Source: three-view drawing plus pictorial views. Frame: mm from the lowest corner of the part. A direction names the side the tool comes from. Give positions to 0.01 mm unless a question says otherwise; leave off trailing zeros. Order: outer loops, then holes, each group sorted by start corner. A loop starts at its lowest first (then second) coordinate and runs counter-clockwise, first axis right, second up. Notation, with made-up numbers: (24.25, 10) -> (83.25, 10) arc R27 cw to (83.25, 28) -> close; hole circle Ø8 at (86, 9.5). An arc over 180 degrees is marked (long way). One line per question, with ' | ' between items.
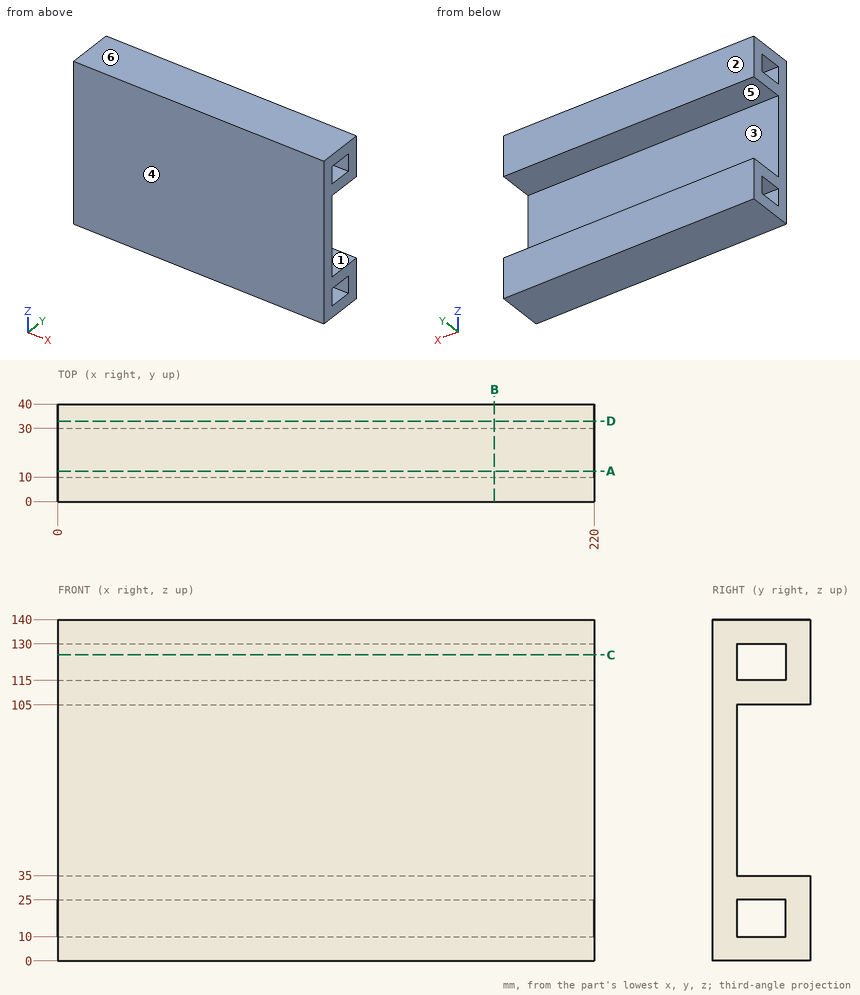
1) Section B-B on x = 179. Return loops of the section in (y, z).
Check result:
outline: (0, 0) -> (40, 0) -> (40, 35) -> (10, 35) -> (10, 105) -> (40, 105) -> (40, 140) -> (0, 140) -> close; hole (10, 10) -> (30, 10) -> (30, 25) -> (10, 25) -> close; hole (10, 115) -> (30, 115) -> (30, 130) -> (10, 130) -> close
2) Section C-C on z = 125.5. Return loops of the section in (x, y), plus the area to 3 significant figures.
Check result:
outline: (0, 0) -> (220, 0) -> (220, 10) -> (0, 10) -> close; (0, 30) -> (220, 30) -> (220, 40) -> (0, 40) -> close | area: 4,400 mm^2
3) Section A-A on y = 12.5. Return loops of the section in (x, z).
Check result:
outline: (0, 0) -> (220, 0) -> (220, 10) -> (0, 10) -> close; (0, 25) -> (220, 25) -> (220, 35) -> (0, 35) -> close; (0, 105) -> (220, 105) -> (220, 115) -> (0, 115) -> close; (0, 130) -> (220, 130) -> (220, 140) -> (0, 140) -> close
4) Section D-D on y = 33. Return loops of the section in (x, z).
Check result:
outline: (0, 0) -> (220, 0) -> (220, 35) -> (0, 35) -> close; (0, 105) -> (220, 105) -> (220, 140) -> (0, 140) -> close
5) Pull-direction query (Z, two-part tool) for the marked faces 3, 4, 5 and 6; classes: +Z half, -Z half, draft (parallel to the pull), parting line (faces both ways), or undercut.
Check result:
face 3: undercut | face 4: draft | face 5: undercut | face 6: +Z half
6) Set-up query: the marked faces 1 and 2. Return all of +Z, -Z, +X, -X, +Y, -Y with unobstructed straight access to the full face (end or side cutting, diameter ignored); none if empty.
Check result:
face 1: +X, -X, +Y | face 2: +Z, -Z, +X, -X, +Y
7) Material intervals for probe 1 along Z at (x, y) = (29, 14); probe 2 along Z at (x, y) = (102, 34); probe 3 along Y at (x, z) = (98, 97), sorted ascending. Write a range as from..to.
Check result:
probe 1: z = 0..10, 25..35, 105..115, 130..140 | probe 2: z = 0..35, 105..140 | probe 3: y = 0..10
8) Contact query for a flat-ended pin moving along its axis: pin 1 Ø16 at (x, y) = (137, 22.5) entering from -Z. Output: stop coordinate, or through.
Check result:
pin 1: stops at z = 0
